Read the model definition and answer for the solid it produces. Units are mm, in the model's axes. Face numbers are marked on the shaded views. Coordinates: 2 decimals unless noted, no trailing zeros. Order: outer loops, then holes, each group sorted by start corner. A loop starts at its lowest first (then second) coordinate and runs counter-clockwise, first axis right, second up. Notation, with made-up numbers: (-11.75, 85.5) - (21.25, 85.5) arc R29 cw to (21.25, 109.5) - close; hole circle Ø4 at (56.25, 74.5). An arc over 180 degrees is marked (long way). Use one line per item in the form item = value.
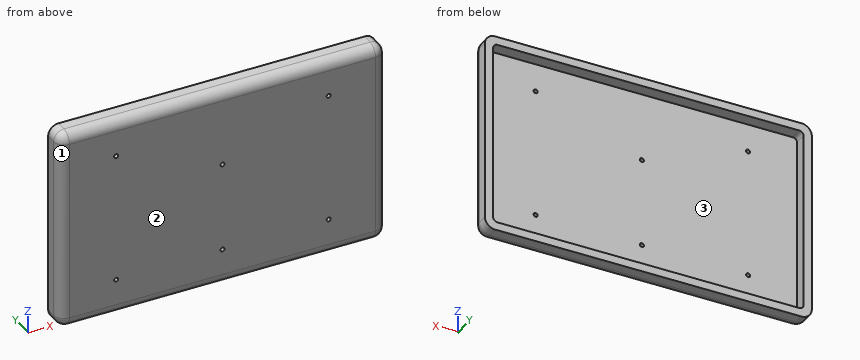
```python
from build123d import *

# Parameters (mm, degrees)
SKETCH1_W             = 200
SKETCH1_H             = 125
BOSS_EXTRUDE1_DEPTH   = 12.7
SKETCH2_W             = 189.84
SKETCH2_H             = 114.84
CUT_EXTRUDE1_DEPTH    = 7.62
FILLET1_R             = 2.54
FILLET2_R             = 6.35
FILLET3_R             = 6.35
M3X0_5_TAPPED_HOLE1_D = 2.5


with BuildPart() as part:
    # Sketch1 → Boss-Extrude1 (new body)
    with BuildSketch(Plane(origin=(0, 0, 0), x_dir=(1, 0, 0), z_dir=(0, 1, 0))):
        Rectangle(SKETCH1_W, SKETCH1_H)
    extrude(amount=BOSS_EXTRUDE1_DEPTH)

    # Sketch2 → Cut-Extrude1 (cut)
    with BuildSketch(Plane(origin=(0, 12.7, 0), x_dir=(1, 0, 0), z_dir=(0, 1, 0))):
        Rectangle(SKETCH2_W, SKETCH2_H)
    extrude(amount=-CUT_EXTRUDE1_DEPTH, mode=Mode.SUBTRACT)

    # Fillet1
    fillet1_edges = [part.edges().sort_by_distance(p)[0] for p in [
        (94.92, 8.89, -57.42),
        (94.92, 8.89, 57.42),
        (-94.92, 8.89, 57.42),
        (-94.92, 8.89, -57.42),
    ]]
    fillet(fillet1_edges, radius=FILLET1_R)

    # Fillet2
    fillet2_edges = [part.edges().sort_by_distance(p)[0] for p in [
        (-100, 6.35, -62.5),
        (100, 6.35, -62.5),
        (100, 6.35, 62.5),
        (-100, 6.35, 62.5),
    ]]
    fillet(fillet2_edges, radius=FILLET2_R)

    # Fillet3
    fillet3_edges = [part.edges().sort_by_distance(p)[0] for p in [
        (0, 0, 62.5),
        (-100, 0, 0),
        (0, 0, -62.5),
        (100, 0, 0),
        (98.140128061, 0, 60.640128061),
        (98.140128061, 0, -60.640128061),
        (-98.140128061, 0, -60.640128061),
        (-98.140128061, 0, 60.640128061),
    ]]
    fillet(fillet3_edges, radius=FILLET3_R)

    # M3x0.5 Tapped Hole1 (through all)
    with Locations(Plane(origin=(0, 5.08, 0), x_dir=(1, 0, 0), z_dir=(0, 1, 0))):
        with Locations((0, -15), (-65, 40), (65, 40), (65, -40), (-65, -40), (0, 40)):
            Hole(M3X0_5_TAPPED_HOLE1_D / 2)


solid = part.part
```
(1) Section A-A, the plane z = 9 is taken. Write down the section's boundary in (x, y), then the cut area to 3 significant figures.
Answer list:
outline = (-100, 6.35) arc R6.35 ccw to (-93.65, 0) - (93.65, 0) arc R6.35 ccw to (100, 6.35) - (100, 12.7) - (94.92, 12.7) - (94.92, 5.08) - (-94.92, 5.08) - (-94.92, 12.7) - (-100, 12.7) - close
area = 1,080 mm2
(2) Section B-B, the plane y = 9.25 is taken. Write down the section's boundary in (x, z), then the cut area to 3 significant figures.
Answer list:
outline = (-100, -56.15) arc R6.35 ccw to (-93.65, -62.5) - (93.65, -62.5) arc R6.35 ccw to (100, -56.15) - (100, 56.15) arc R6.35 ccw to (93.65, 62.5) - (-93.65, 62.5) arc R6.35 ccw to (-100, 56.15) - close; hole (-94.92, -54.88) arc R2.54 ccw to (-92.38, -57.42) - (92.38, -57.42) arc R2.54 ccw to (94.92, -54.88) - (94.92, 54.88) arc R2.54 ccw to (92.38, 57.42) - (-92.38, 57.42) arc R2.54 ccw to (-94.92, 54.88) - close
area = 3,170 mm2
(3) Straight lines are drawn through the part: L1, parallel to Z at x = -27.5, y = 12.25; L2, parallel to X at y = 2.85, z = -40; L3, parallel to X at y = 9.75, z = 39. For each, find the intervals that lie inside material, in ascending order.
Answer list:
L1 = -62.5 to -57.42, 57.42 to 62.5
L2 = -98.95 to -66.25, -63.75 to -1.25, 1.25 to 63.75, 66.25 to 98.95
L3 = -100 to -94.92, 94.92 to 100
(4) Given pin 1 Ø3 at (x, z) = (0, -40) entering from +Y; pin 2 Ø1.5 at (x, y) = (-78, 2.5) entering from -Z; pin 3 Ø1.5 at (y, z) = (3, -43) entering from +X, each flat-ended and moving along its own axis, determine where each tip first touches the part or whether it passes through.
Answer list:
pin_1 = 5.08
pin_2 = -61.69
pin_3 = 99.44
(5) Section C-C, the plane x = 60 is taken. Write down the section's boundary in (y, z), then the cut area to 3 significant figures.
Answer list:
outline = (0, -56.15) arc R6.35 ccw to (6.35, -62.5) - (12.7, -62.5) - (12.7, -57.42) - (5.08, -57.42) - (5.08, 57.42) - (12.7, 57.42) - (12.7, 62.5) - (6.35, 62.5) arc R6.35 ccw to (0, 56.15) - close
area = 695 mm2
(6) The mould has two halves that part along X. Classify the marked faces 1, 2 and 3: +X half, -X half, draft (parallel to the pull), parting line (faces both ways), or undercut.
Answer list:
face_1 = -X half
face_2 = draft
face_3 = undercut
